For this review, take the finished solid that the model builds, in its own axes (mm). A direction names the side the tool comes from. Coordinates: 2 decimals unless noted, no trailing zeros. Loops run counter-clockwise (first coordinate to the right, second up) from the corner with the lowest first, then second, coordinate; pieces in that order, holes last. Notation, with made-up numbers: M 74.5,85 L 113.5,85 A19 ccw 113.5,98 Z; hole C -30.75,0 d7. An arc over 180 degrees is marked long. Answer as a JSON object with one key per item and string values. Group by question number.
Item 1: Add section B-B (x = 34). State the section outline as (y, z) points.
Item 2: Add section A-A (y = 17). State the section outline as (x, z) points, then the cut area to 3 significant figures.
Item 3: Mouldability with a two-part tool opening along X and no side actions: class faces 3 (the face through (35.6, 0.99, -15.67)), 4 (the face through (50.3, 1.01, 17.94)), 5 (the face through (1, 21, -6.6)) as +X half, -X half, draft (parallel to the pull), parting line (faces both ways), or undercut.
Item 4: Wall thickness on L1, parallel to Z at x = 40.4, y = 1.15; L2, parallel to X at y = 28, z = -10.5: over which ranges is each line inside the solid? List them lowest first. Write a range as from..to.
Item 5: Add section C-C (z = -4). State the section outline as (x, y) points.
Item 6: Add section D-D (x = 25). State the section outline as (y, z) points.
Item 7: Tool access review of faces 1 (the face through (35.6, 0.99, 15.53)), 2 (the face through (1, 7.2, 0.1)): name each direction out of +Z, -Z, +X, -X, +Y, -Y from which nothing blocks a thin tool from reaching the whole face with its end or side.
Item 8: Insertion check: pin 1 (3.5 mm diameter, centred on x = 21.2, z = -15.6, fed in from +Y); pin 2 (2 mm diameter, centred on y = 12.5, z = 6, fed in from +X); pin 3 (1.6 mm diameter, centred on x = 1, y = 22, fed in from -Z). Each pin has a flat end and moves straight along its axis. Give the tip position at first contact, or say it passes through.
from build123d import *

# Parameters (mm, degrees)
BOSS_EXTRUDE1_DEPTH            = 18.8
CUT_EXTRUDE1_START             = -2
SKETCH2_R                      = 1.204354552
CUT_EXTRUDE1_DEPTH             = 2
FILLET1_R                      = 3
F_3_2_3_2_DIAMETER_HOLE1_D     = 3.2
F_3_2_3_2_DIAMETER_HOLE1_DEPTH = 2


with BuildPart() as part:
    # Sketch1 → Boss-Extrude1 (new body, symmetric)
    with BuildSketch(Plane.XY):
        with BuildLine():
            Line((2.5, 0), (51.2, 0))
            Line((51.2, 0), (51.2, 2))
            Line((51.2, 2), (3, 2))
            ThreePointArc((3, 2), (2.292893219, 2.292893219), (2, 3))
            Line((2, 3), (2, 39.6))
            Line((2, 39.6), (0, 39.6))
            Line((0, 39.6), (0, 2.5))
            ThreePointArc((0, 2.5), (0.732233047, 0.732233047), (2.5, 0))
        make_face()
    extrude(amount=BOSS_EXTRUDE1_DEPTH, both=True)

    # Sketch2 → Cut-Extrude1 (cut)
    with BuildSketch(Plane.ZY.offset(CUT_EXTRUDE1_START)):
        with Locations((15.5, 20.8)):
            Circle(SKETCH2_R)
        with Locations((7.75, 7.376606241)):
            Circle(SKETCH2_R)
        with Locations((-7.75, 7.376606241)):
            Circle(SKETCH2_R)
        with Locations((-15.5, 20.8)):
            Circle(SKETCH2_R)
        with Locations((-7.75, 34.223393759)):
            Circle(SKETCH2_R)
        with Locations((7.75, 34.223393759)):
            Circle(SKETCH2_R)
        with BuildLine():
            Line((6.6, 27.8), (6.6, 13.8))
            ThreePointArc((6.6, 13.8), (0, 7.2), (-6.6, 13.8))
            Line((-6.6, 13.8), (-6.6, 27.8))
            ThreePointArc((-6.6, 27.8), (0, 34.4), (6.6, 27.8))
        make_face()
        with BuildLine():
            Line((-18.8, 40.1), (-18.8, 20.8))
            ThreePointArc((-18.8, 20.8), (0, 39.6), (18.8, 20.8))
            Line((18.8, 20.8), (18.8, 40.1))
            Line((18.8, 40.1), (-18.8, 40.1))
        make_face()
    extrude(amount=CUT_EXTRUDE1_DEPTH, mode=Mode.SUBTRACT)

    # Fillet1
    fillet1_edges = [part.edges().sort_by_distance(p)[0] for p in [
        (51.2, 1, -18.8),
        (51.2, 1, 18.8),
    ]]
    fillet(fillet1_edges, radius=FILLET1_R)

    # Ø3.2 (3.2) Diameter Hole1
    with Locations(Plane(origin=(0, 2, 0), x_dir=(1, 0, 0), z_dir=(0, 1, 0))):
        with Locations((8.4, 15.6), (8.4, -15.6), (14.8, 15.6), (14.8, -15.6), (21.2, 15.6), (21.2, -15.6), (27.6, 15.6), (27.6, -15.6), (34, 15.6), (34, -15.6), (40.4, 15.6), (40.4, -15.6), (46.8, 15.6), (46.8, -15.6)):
            Hole(F_3_2_3_2_DIAMETER_HOLE1_D / 2, depth=F_3_2_3_2_DIAMETER_HOLE1_DEPTH)


solid = part.part
From the geometry:
{
 "1": {"outline": "M 0,-18.8 L 2,-18.8 L 2,-17.2 L 0,-17.2 Z; M 0,-14 L 2,-14 L 2,14 L 0,14 Z; M 0,17.2 L 2,17.2 L 2,18.8 L 0,18.8 Z"},
 "2": {"outline": "M 0,-18.8 L 2,-18.8 L 2,-6.6 L 0,-6.6 Z; M 0,6.6 L 2,6.6 L 2,18.8 L 0,18.8 Z", "area": "48.8 mm²"},
 "3": {"face 3": "undercut", "face 4": "+X half", "face 5": "draft"},
 "4": {"L1": "z = -18.8..-17.2, -14..14, 17.2..18.8", "L2": "x = 0..2"},
 "5": {"outline": "M 0,2.5 A2.5 ccw 2.5,0 L 51.2,0 L 51.2,2 L 3,2 A1 cw 2,3 L 2,8.55 L 0,8.55 Z; M 0,33.05 L 2,33.05 L 2,39.17 L 0,39.17 Z"},
 "6": {"outline": "M 0,-18.8 L 2,-18.8 L 2,18.8 L 0,18.8 Z"},
 "7": {"face 1": "+Y, -Y", "face 2": "+X, -X"},
 "8": {"pin 1": "stops at y = 2", "pin 2": "stops at x = 2", "pin 3": "stops at z = -18.8"}
}
